Model file for the job. Use its own axes, mm. A direction names the side the tool comes from. Round coordinates to 2 decimals unless told otherwise and drop trailing zeros. Write item = value, one per line.
```python
from build123d import *

# Parameters (mm, degrees)
SKETCH1_W               = 130.048
SKETCH1_H               = 152.4
BOSS_EXTRUDE1_DEPTH     = 2.54
CHAMFER1_SIZE           = 2.54
SKETCH4_W               = 6.35
SKETCH4_H               = 12.7
BOSS_EXTRUDE4_DEPTH     = 25.4
CUT_EXTRUDE2_DEPTH      = 104.996173853
CUT_EXTRUDE2_DEPTH_BACK = 104.996173853
SKETCH5_R               = 2.667
CUT_EXTRUDE3_DEPTH      = 60.452
CUT_EXTRUDE3_DEPTH_BACK = 60.452
SKETCH5_3_R             = 2.667
FILLET1_R               = 7.62
FILLET2_R               = 2.54
CHAMFER2_SIZE           = 2.54
SKETCH6_R               = 1.905
CUT_EXTRUDE4_DEPTH      = 104.996173853
SKETCH8_R               = 1.905
CUT_EXTRUDE5_DEPTH      = 2.54
SKETCH9_R               = 1.905
CUT_EXTRUDE6_DEPTH      = 104.996173853
CUT_EXTRUDE7_DEPTH      = 104.996173853
FILLET3_R               = 2.54


with BuildPart() as part:
    # Sketch1 → Boss-Extrude1 (new body)
    with BuildSketch(Plane(origin=(0, 0, 0), x_dir=(1, 0, 0), z_dir=(0, 1, 0))):
        Rectangle(SKETCH1_W, SKETCH1_H)
    extrude(amount=BOSS_EXTRUDE1_DEPTH)

    # Chamfer1
    chamfer1_edges = [part.edges().sort_by_distance(p)[0] for p in [
        (0, 0, -76.2),
        (-65.024, 0, 0),
        (0, 0, 76.2),
        (65.024, 0, 0),
    ]]
    chamfer(chamfer1_edges, length=CHAMFER1_SIZE - 0.0001)  # a hair under: the kernel refuses the full size

    # Sketch4 → Boss-Extrude4 (add)
    with BuildSketch(Plane(origin=(0, 2.54, 0), x_dir=(1, 0, 0), z_dir=(0, 1, 0))):
        with Locations((-58.547, 66.548)):
            Rectangle(SKETCH4_W, SKETCH4_H)
        with Locations((-58.547, 0)):
            Rectangle(SKETCH4_W, SKETCH4_H)
        with Locations((-58.547, -66.548)):
            Rectangle(SKETCH4_W, SKETCH4_H)
        with Locations((58.547, -66.548)):
            Rectangle(SKETCH4_W, SKETCH4_H)
        with Locations((58.547, 0)):
            Rectangle(SKETCH4_W, SKETCH4_H)
        with Locations((58.547, 66.548)):
            Rectangle(SKETCH4_W, SKETCH4_H)
    extrude(amount=BOSS_EXTRUDE4_DEPTH)

    # Sketch5 → Cut-Extrude2 (cut, two sides: drawn at the far end of the back side and taken through both)
    with BuildSketch(Plane(origin=(0, 0, 0), x_dir=(0, 0, -1), z_dir=(1, 0, 0)).offset(-CUT_EXTRUDE2_DEPTH_BACK)):
        with Locations((-66.548, 21.59)):
            Circle(SKETCH5_R)
        with Locations((0, 21.59)):
            Circle(SKETCH5_R)
        with Locations((66.548, 21.59)):
            Circle(SKETCH5_R)
    extrude(amount=CUT_EXTRUDE2_DEPTH + CUT_EXTRUDE2_DEPTH_BACK, mode=Mode.SUBTRACT)

    # Sketch5<3> → Cut-Extrude3 (cut, two sides: drawn at the far end of the back side and taken through both)
    # profile 1 of 3: a face of its own
    with BuildSketch(Plane(origin=(0, 0, 0), x_dir=(0, 0, -1), z_dir=(1, 0, 0)).offset(-CUT_EXTRUDE3_DEPTH_BACK)):
        Polygon((0, 16.823973528), (4.1275, 19.206986764), (4.1275, 23.973013236), (0, 26.356026472), (-4.1275, 23.973013236), (-4.1275, 19.206986764), align=None)
        with Locations(Location((0, 21.59, 0), (0, 0, 180))):
            Circle(SKETCH5_3_R, mode=Mode.SUBTRACT)
    # profile 2 of 3: a face of its own
    with BuildSketch(Plane(origin=(0, 0, 0), x_dir=(0, 0, -1), z_dir=(1, 0, 0)).offset(-CUT_EXTRUDE3_DEPTH_BACK)):
        Polygon((-66.548, 16.823973528), (-62.4205, 19.206986764), (-62.4205, 23.973013236), (-66.548, 26.356026472), (-70.6755, 23.973013236), (-70.6755, 19.206986764), align=None)
        with Locations(Location((-66.548, 21.59, 0), (0, 0, 180))):
            Circle(SKETCH5_3_R, mode=Mode.SUBTRACT)
    # profile 3 of 3: a face of its own
    with BuildSketch(Plane(origin=(0, 0, 0), x_dir=(0, 0, -1), z_dir=(1, 0, 0)).offset(-CUT_EXTRUDE3_DEPTH_BACK)):
        Polygon((66.548, 16.823973528), (70.6755, 19.206986764), (70.6755, 23.973013236), (66.548, 26.356026472), (62.4205, 23.973013236), (62.4205, 19.206986764), align=None)
        with Locations(Location((66.548, 21.59, 0), (0, 0, 180))):
            Circle(SKETCH5_3_R, mode=Mode.SUBTRACT)
    extrude(amount=CUT_EXTRUDE3_DEPTH + CUT_EXTRUDE3_DEPTH_BACK, mode=Mode.SUBTRACT)

    # Fillet1
    fillet1_edges = [part.edges().sort_by_distance(p)[0] for p in [
        (-58.547, 2.54, -60.198),
        (-58.547, 2.54, 6.35),
        (-58.547, 2.54, -6.35),
        (-58.547, 2.54, 60.198),
        (58.547, 2.54, 60.198),
        (58.547, 2.54, -6.35),
        (58.547, 2.54, 6.35),
        (58.547, 2.54, -60.198),
    ]]
    fillet(fillet1_edges, radius=FILLET1_R)

    # Fillet2
    fillet2_edges = [part.edges().sort_by_distance(p)[0] for p in [
        (-55.372, 2.54, -62.738),
        (-55.372, 2.54, 0),
        (-55.372, 2.54, 62.738),
        (55.372, 2.54, 62.738),
        (55.372, 2.54, 0),
        (55.372, 2.54, -62.738),
    ]]
    fillet(fillet2_edges, radius=FILLET2_R)

    # Chamfer2
    chamfer2_edges = [part.edges().sort_by_distance(p)[0] for p in [
        (-58.547, 27.94, -60.198),
        (-58.547, 27.94, -72.898),
        (-58.547, 27.94, 6.35),
        (-58.547, 27.94, -6.35),
        (-58.547, 27.94, 72.898),
        (-58.547, 27.94, 60.198),
        (58.547, 27.94, 60.198),
        (58.547, 27.94, 72.898),
        (58.547, 27.94, -6.35),
        (58.547, 27.94, 6.35),
        (58.547, 27.94, -72.898),
        (58.547, 27.94, -60.198),
    ]]
    chamfer(chamfer2_edges, length=CHAMFER2_SIZE)

    # Sketch6 → Cut-Extrude4 (cut, through all)
    with BuildSketch(Plane.XZ):
        with Locations(Location((26.035, 58.42, 0), (0, 0, 270))):
            Circle(SKETCH6_R)
        with Locations(Location((24.765, 12.7, 0), (0, 0, 270))):
            Circle(SKETCH6_R)
        with Locations(Location((-26.035, 55.88, 0), (0, 0, 270))):
            Circle(SKETCH6_R)
        with Locations(Location((-26.035, 27.94, 0), (0, 0, 270))):
            Circle(SKETCH6_R)
    extrude(amount=-CUT_EXTRUDE4_DEPTH, mode=Mode.SUBTRACT)

    # Sketch8 → Cut-Extrude5 (cut)
    with BuildSketch(Plane.XZ):
        with Locations(Location((29, -12.33, 0), (0, 0, 270))):
            Circle(SKETCH8_R)
        with Locations(Location((29, -61.33, 0), (0, 0, 270))):
            Circle(SKETCH8_R)
        with Locations(Location((-29, -61.33, 0), (0, 0, 270))):
            Circle(SKETCH8_R)
        with Locations(Location((-29, -12.33, 0), (0, 0, 270))):
            Circle(SKETCH8_R)
    extrude(amount=-CUT_EXTRUDE5_DEPTH, mode=Mode.SUBTRACT)

    # Sketch9 → Cut-Extrude6 (cut, through all)
    with BuildSketch(Plane.XZ):
        with Locations(Location((-49.784, -69.85, 0), (0, 0, 270))):
            Circle(SKETCH9_R)
        with Locations(Location((-49.784, 69.85, 0), (0, 0, 270))):
            Circle(SKETCH9_R)
        with Locations(Location((49.784, 69.85, 0), (0, 0, 270))):
            Circle(SKETCH9_R)
        with Locations(Location((49.784, -69.85, 0), (0, 0, 270))):
            Circle(SKETCH9_R)
    extrude(amount=-CUT_EXTRUDE6_DEPTH, mode=Mode.SUBTRACT)

    # Sketch10 → Cut-Extrude7 (cut, through all)
    with BuildSketch(Plane.XZ):
        with BuildLine():
            Line((-6.35, -19.05), (-6.35, 19.05))
            ThreePointArc((-6.35, 19.05), (0, 25.4), (6.35, 19.05))
            Line((6.35, 19.05), (6.35, -19.05))
            ThreePointArc((6.35, -19.05), (0, -25.4), (-6.35, -19.05))
        make_face()
    extrude(amount=-CUT_EXTRUDE7_DEPTH, mode=Mode.SUBTRACT)

    # Fillet3
    fillet3_edges = [part.edges().sort_by_distance(p)[0] for p in [
        (0, 2.54, 25.4),
        (6.35, 2.54, 0),
        (0, 2.54, -25.4),
        (-6.35, 2.54, 0),
    ]]
    fillet(fillet3_edges, radius=FILLET3_R - 0.0001)  # a hair under: the kernel refuses the full size


solid = part.part
```
1) 3-axis set-ups, long thin cutter, end or side, ignore diameter. For faces 1 (the face through (57.88, 18.03, 68.64)), 2 (the face through (-59, 18, 60.198)), 3 (the face through (-55.372, 14, 66)): which of +Z, -Z, +X, -X, +Y, -Y reach the whole face in a straight line?
Conclusion:
face_1 = none
face_2 = +X, -X, +Y
face_3 = +Z, -Z, +Y
2) Mould opens along X. For faces 4 (the face through (61.722, 15, -65)), 5 (the face through (-60.452, 19.5, 1.9)), 6 (the face through (59, 27.94, -67)) say: +X half, -X half, draft (parallel to the pull), parting line (faces both ways), or undercut.
Conclusion:
face_4 = +X half
face_5 = undercut
face_6 = draft
3) Wall check: line 1 along Z through (x, y) = (61.2, 21.59) (3 decimals); line 2 along Y through (x, z) = (61.35, 0); line 3 along X through (y, z) = (17.75, -62). Give the ranges that are in metal, low to high.
Conclusion:
line_1 = -72.898 to -69.215, -63.881 to -60.198, -6.35 to -2.667, 2.667 to 6.35, 60.198 to 63.881, 69.215 to 72.898
line_2 = 0 to 18.92, 24.26 to 27.94
line_3 = -61.72 to -55.37, 55.37 to 61.72
4) Flat gauge pins, fed straight in: pin 1 Ø5 at (x, y) = (58.5, 19.5) entering from -Z; pin 2 Ø6 at (x, z) = (24.765, 12.7) entering from +Y; pin 3 Ø4.5 at (x, y) = (55.5, 11.5) entering from +Z; pin 4 Ø5 at (y, z) = (21.59, -66.548) entering from +X. Where does each tip first touch, or does it go through?
Conclusion:
pin_1 = -72.9
pin_2 = 2.54
pin_3 = 72.9
pin_4 = through
